Part print with two shaded views. Sizes in mm from the minimum x, y, z corner. A direction names the side the tool comes from. Coordinates: 2 decimals unless noted, no trailing zeros. Order: outer loops, then holes, each group sorted by start corner. A loop starts at its lowest first (then second) coordinate and runs counter-clockwise, first axis right, second up. Notation, with made-up numbers: (63, 76) - (120, 76) arc R17 cw to (120, 94) - close; hole circle Ø4 at (30.5, 10.5). An arc over 180 degrees is marked (long way). Write each question's results on one line, items separated by ' | '. Start each with the question number.
Q1. Which spindle directions (+Z, -Z, +X, -X, +Y, -Y) get a long thin tool onto all of the face, cutting with end or side? Do the marked faces 5, 6, 7 and 8. Say none if no direction does.
Q2. Wall check: probe 1 along Z at (x, y) = (25.75, 4.75); probe 2 along X at (y, z) = (10, 9.5); probe 3 along Y at (x, z) = (14.6, 18). Give the ranges that are in metal, low to high.
Q3. Band-saw the part on D-D, the plane y = 11. Write the cut outline in (x, z), then the cut area to 3 significant figures.
Q4. Pin check, flat tips, straight feed: P1, Ø3.5, axis at x = 3, y = 2.5, coming from the -Z side; P2, Ø6, axis at y = 13, z = 30, coming from the +X side; P3, Ø2.5, axis at x = 24, y = 19.5, coming from the +Z side; P4, Ø4.5, axis at x = 13, z = 24.5, coming from the +Y side. Stop position of each tip, or through.
Q5. Band-saw the part on C-C, the plane y = 19.5. Write the cut outline in (x, z), then the cut area to 4 significant figures.
Q6. Band-saw the part on B-B, the plane z = 18. Write the cut outline in (x, y), then the cut area to 3 significant figures.
Q7. Pull direction Y, two halves, no side cores. Call the marked faces 1, 2, 3 and 4: released by +Y, released by -Y, zero draft, split by the parting line, or undercut.
Q8. Band-saw the part on A-A, the plane x = 24. Write the cut outline in (y, z), then the cut area to 3 significant figures.
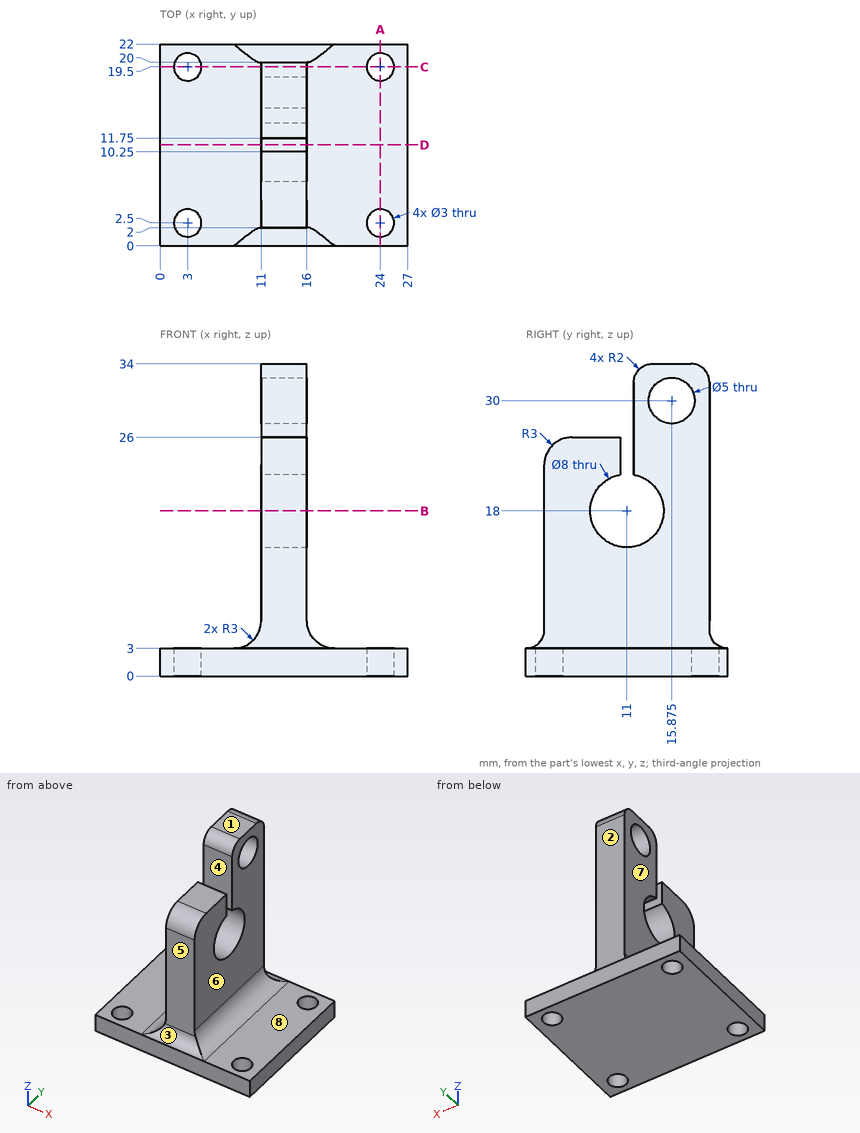
Results below:
1) face 5: +Z, +X, -X, -Y | face 6: +Z, +X, +Y, -Y | face 7: +Z, -X, +Y, -Y | face 8: +Z, +X, +Y, -Y
2) probe 1: z = 0 to 3 | probe 2: x = 11 to 16 | probe 3: y = 2 to 7, 15 to 20
3) outline: (0, 0) - (27, 0) - (27, 3) - (19, 3) arc R3 cw to (16, 6) - (16, 14) - (11, 14) - (11, 6) arc R3 cw to (8, 3) - (0, 3) - close | area: 140 mm²
4) P1: stops at z = 0 | P2: stops at x = 16 | P3: passes through | P4: stops at y = 20
5) outline: (0, 0) - (1.5, 0) - (1.5, 3) - (0, 3) - close; (4.5, 0) - (22.5, 0) - (22.5, 3) - (19, 3) arc R3 cw to (16, 6) - (16, 33.32) - (11, 33.32) - (11, 6) arc R3 cw to (8, 3) - (4.5, 3) - close; (25.5, 0) - (27, 0) - (27, 3) - (25.5, 3) - close | area: 218.5 mm²
6) outline: (11, 2) - (16, 2) - (16, 7) - (11, 7) - close; (11, 15) - (16, 15) - (16, 20) - (11, 20) - close | area: 50.0 mm²
7) face 1: zero draft | face 2: released by +Y | face 3: released by -Y | face 4: undercut
8) outline: (0, 0) - (1, 0) - (1, 3) - (0, 3) - close; (4, 0) - (18, 0) - (18, 3) - (4, 3) - close; (21, 0) - (22, 0) - (22, 3) - (21, 3) - close | area: 48.0 mm²
